Input: part model. Units: mm. Frame: model coordinates. A direction names the side the tool comes from. Coordinates: 2 decimals unless noted, no trailing zeros. Loops run counter-clockwise (first coordinate to the right, second up) from the corner with the lowest first, then second, coordinate; pieces in that order, holes last.
(1) Line query: L1, parallel to X at y = 3.25, z = 0; L2, parallel to X at y = 4, z = -31.5; L3, parallel to Z at x = 96.5, y = -6.75. Output: solid intervals per line, ascending.
(2) Mould query, pull axis Z, two halves, no side actions, for faces 3 (the face through (186, 9.5, 17)), 4 (the face through (137.02, -0.13, 87.36)), 5 (the face through (10.99, 0.13, -249.76)). Classes: released by +Z, released by -Z, zero draft, split by the parting line, or undercut.
(3) Contact query for flat-ended pins moving along their axis: P1, Ø11.5, axis at x = -111.25, z = 192.69, coming from the -Y side; P2, Ø5, axis at y = 3, z = -193.5, coming from the -X side; P3, Ø4, axis at y = 1, z = 156, coming from the -X side; P4, Ø8, axis at y = 7, z = 23, coming from the -X side. Output: stop coordinate, or through.
(4) Section B-B, the plane x = 0. Return loops of the section in (y, z), then the cut area to 3 significant figures.
(5) Set-up query: faces 1 (the face through (116.246, 6.542, -126.771)), 2 (the face through (103, 9.5, 127)). Return all of +Z, -Z, +X, -X, +Y, -Y with unobstructed straight access to the full face (end or side cutting, diameter ignored); none if empty.
(6) Section A-A, the plane y = -2.25. Return loops of the section in (x, z), then the cut area to 3 significant figures.
(7) Section C-C, the plane z = -123. Return loops of the section in (x, y), then the cut area to 3 significant figures.
```python
from build123d import *

# Parameters (mm, degrees)
SKETCH1_R           = 250
SKETCH1_R_2         = 162.5
BOSS_EXTRUDE1_DEPTH = 9.5
SKETCH2_R           = 5
CUT_EXTRUDE1_DEPTH  = 355.063553617
SKETCH3_R           = 183
SKETCH3_R_2         = 172
CUT_EXTRUDE2_DEPTH  = 6


with BuildPart() as part:
    # Sketch1 → Boss-Extrude1 (new, symmetric)
    with BuildSketch(Plane(origin=(0, 0, 0), x_dir=(1, 0, 0), z_dir=(0, 1, 0))):
        with Locations(Location((0, 0, 0), (0, 0, 270))):
            Circle(SKETCH1_R)
        with Locations(Location((0, 0, 0), (0, 0, 270))):
            Circle(SKETCH1_R_2, mode=Mode.SUBTRACT)
    extrude(amount=BOSS_EXTRUDE1_DEPTH, both=True)

    # Sketch2 → Cut-Extrude1 (cut, through all)
    with BuildSketch(Plane(origin=(0, 9.5, 0), x_dir=(1, 0, 0), z_dir=(0, 1, 0))):
        with Locations(Location((111.25, 192.690652342, 0), (0, 0, 270))):
            Circle(SKETCH2_R)
        with Locations(Location((222.5, 0, 0), (0, 0, 270))):
            Circle(SKETCH2_R)
        with Locations(Location((-222.5, 0, 0), (0, 0, 90))):
            Circle(SKETCH2_R)
        with Locations(Location((-111.25, 192.690652342, 0), (0, 0, 90))):
            Circle(SKETCH2_R)
        with Locations(Location((111.25, -192.690652342, 0), (0, 0, 90))):
            Circle(SKETCH2_R)
        with Locations(Location((-111.25, -192.690652342, 0), (0, 0, 270))):
            Circle(SKETCH2_R)
    extrude(amount=-CUT_EXTRUDE1_DEPTH, mode=Mode.SUBTRACT)

    # Sketch3 → Cut-Extrude2 (cut)
    with BuildSketch(Plane(origin=(0, 9.5, 0), x_dir=(1, 0, 0), z_dir=(0, 1, 0))):
        with Locations(Location((0, 0, 0), (0, 0, 270))):
            Circle(SKETCH3_R)
        with Locations(Location((0, 0, 0), (0, 0, 270))):
            Circle(SKETCH3_R_2, mode=Mode.SUBTRACT)
    extrude(amount=-CUT_EXTRUDE2_DEPTH, mode=Mode.SUBTRACT)


solid = part.part
```
Report:
1. L1: x = -250 to -227.5, -217.5 to -162.5, 162.5 to 217.5, 227.5 to 250
1. L2: x = -248.01 to -180.27, -169.09 to -159.42, 159.42 to 169.09, 180.27 to 248.01
1. L3: z = -230.62 to -130.74, 130.74 to 230.62
2. face 3: zero draft
2. face 4: undercut
2. face 5: split by the parting line
3. P1: stops at y = -9.5
3. P2: stops at x = -161.3
3. P3: stops at x = -196.94
3. P4: stops at x = -249.28
4. outline: (-9.5, -250) - (9.5, -250) - (9.5, -183) - (3.5, -183) - (3.5, -172) - (9.5, -172) - (9.5, -162.5) - (-9.5, -162.5) - close; (-9.5, 162.5) - (9.5, 162.5) - (9.5, 172) - (3.5, 172) - (3.5, 183) - (9.5, 183) - (9.5, 250) - (-9.5, 250) - close
4. area: 3,190 mm2
5. face 1: +Y
5. face 2: +Z, -Z, +X, -X, +Y
6. outline: circle Ø500 at (0, 0); hole circle Ø10 at (-222.5, 0); hole circle Ø325 at (0, 0); hole circle Ø10 at (-111.25, -192.69); hole circle Ø10 at (-111.25, 192.69); hole circle Ø10 at (111.25, -192.69); hole circle Ø10 at (111.25, 192.69); hole circle Ø10 at (222.5, 0)
6. area: 113,000 mm2
7. outline: (-217.65, -9.5) - (-106.19, -9.5) - (-106.19, 9.5) - (-120.23, 9.5) - (-120.23, 3.5) - (-135.5, 3.5) - (-135.5, 9.5) - (-217.65, 9.5) - close; (106.19, -9.5) - (217.65, -9.5) - (217.65, 9.5) - (135.5, 9.5) - (135.5, 3.5) - (120.23, 3.5) - (120.23, 9.5) - (106.19, 9.5) - close
7. area: 4,050 mm2
